The listing builds one solid part. Answer for the finished solid, in the listing's coordinates (mm). Face numbers are marked on the shaded views. A direction names the side the tool comes from. Round coordinates to 2 decimals unless told otherwise and drop trailing zeros. Loops run counter-clockwise (first coordinate to the right, second up) from the corner with the lowest first, then second, coordinate; pieces in that order, holes last. Notation, with made-up numbers: (81.5, 54.5) - (102.5, 54.5) arc R16 cw to (102.5, 79.5) - close; hole circle Ø1 at (-25, 82.25). An arc over 180 degrees is marked (long way). One line per item, written item: value.
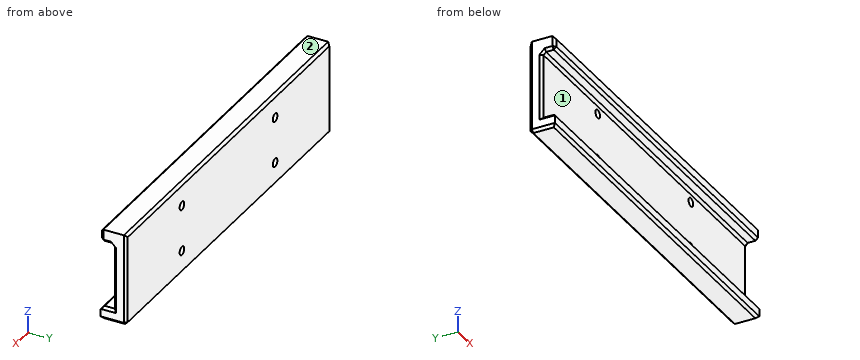
```python
from build123d import *

# Parameters (mm, degrees)
SKETCH1_W                       = 147
SKETCH1_H                       = 36
BOSS_EXTRUDE1_DEPTH             = 5
SKETCH2_W                       = 26
SKETCH2_H                       = 5
CUT_EXTRUDE1_DEPTH              = 74.5
CUT_EXTRUDE1_DEPTH_BACK         = 74.5
CHAMFER1_SIZE                   = 1
TAP_DRILL_FOR_M4X0_7_TAP1_D     = 3.3
TAP_DRILL_FOR_M4X0_7_TAP1_DEPTH = 14
TAP_DRILL_FOR_M4X0_7_TAP1_TIP   = 0.991420021


with BuildPart() as part:
    # Sketch1 → Boss-Extrude1 (new body, symmetric)
    with BuildSketch(Plane(origin=(0, 0, 0), x_dir=(1, 0, 0), z_dir=(0, 1, 0))):
        Rectangle(SKETCH1_W, SKETCH1_H)
    extrude(amount=BOSS_EXTRUDE1_DEPTH, both=True)

    # Sketch2 → Cut-Extrude1 (cut, two sides)
    with BuildSketch(Plane(origin=(0, 0, 0), x_dir=(0, 0, -1), z_dir=(1, 0, 0))) as cut_extrude1_sk:
        with Locations((0, -2.5)):
            Rectangle(SKETCH2_W, SKETCH2_H)
    extrude(amount=CUT_EXTRUDE1_DEPTH, mode=Mode.SUBTRACT)
    extrude(cut_extrude1_sk.sketch, amount=-CUT_EXTRUDE1_DEPTH_BACK, mode=Mode.SUBTRACT)

    # Chamfer1
    chamfer1_edges = [part.edges().sort_by_distance(p)[0] for p in [
        (73.5, -2.5, 13),
        (0, -5, 18),
        (0, 0, 13),
        (73.5, 0, 0),
        (73.5, -2.5, -13),
        (0, -5, -13),
        (-73.5, -2.5, -13),
        (-73.5, 0, 0),
        (-73.5, -2.5, 13),
        (-73.5, -5, 15.5),
        (0, -5, 13),
        (73.5, -5, 15.5),
        (0, 5, 18),
        (-73.5, 5, 0),
        (73.5, 5, 0),
        (0, 5, -18),
        (73.5, 0, -18),
        (0, -5, -18),
        (-73.5, 0, -18),
    ]]
    chamfer(chamfer1_edges, length=CHAMFER1_SIZE)

    # Tap Drill for M4x0.7 Tap1
    with Locations(Plane(origin=(-88.5, 5, -18), x_dir=(-1, 0, 0), z_dir=(0, 1, 0))):
        with Locations((-55, 27), (-122, 27), (-55, 9), (-122, 9)):
            Hole(TAP_DRILL_FOR_M4X0_7_TAP1_D / 2, depth=TAP_DRILL_FOR_M4X0_7_TAP1_DEPTH)
            with Locations((0, 0, -(TAP_DRILL_FOR_M4X0_7_TAP1_DEPTH + TAP_DRILL_FOR_M4X0_7_TAP1_TIP / 2))):  # 118° drill point
                Cone(0, TAP_DRILL_FOR_M4X0_7_TAP1_D / 2, TAP_DRILL_FOR_M4X0_7_TAP1_TIP, mode=Mode.SUBTRACT)


solid = part.part
```
1) For the marked faces 1 and 2, determine the directions among +Z, -Z, +X, -X, +Y, -Y from which every point of the face is accessible in a straight line to the end or side of a thin tool.
Final values:
face 1: +X, -X, -Y
face 2: +Z, +X, -X, +Y, -Y
2) Each of these flat-tipped pins is pushed along its axis until it touches: pin 1 Ø2.5 at (x, z) = (33.5, 9) entering from +Y; pin 2 Ø4 at (x, z) = (-33.5, -9) entering from -Y. Where does it stop, or does it pass through?
Final values:
pin 1: through
pin 2: y = 0
3) A cutting plane is placed at A-A on z = -9. Give the vertices of the cut face in (x, y).
Final values:
outline: (-73.5, 1) - (-72.5, 0) - (-35.15, 0) - (-35.15, 5) - (-72.5, 5) - (-73.5, 4) - close; (-31.85, 0) - (31.85, 0) - (31.85, 5) - (-31.85, 5) - close; (35.15, 0) - (72.5, 0) - (73.5, 1) - (73.5, 4) - (72.5, 5) - (35.15, 5) - close
4) Consider L1, parallel to Z at x = -33.5, y = 3; L2, parallel to Z at x = 54, y = -1.75; L3, parallel to Y at x = -49.5, z = -6.5. Determine where each line is inside the solid, lowest interval first.
Final values:
L1: -18 to -10.65, -7.35 to 7.35, 10.65 to 18
L2: -18 to -13, 13 to 18
L3: 0 to 5
5) A cutting plane is placed at B-B on x = -33.5. Give the vertices of the cut face in (y, z).
Final values:
outline: (-5, -17) - (-4, -18) - (4, -18) - (5, -17) - (5, -10.65) - (0, -10.65) - (0, -13) - (-4, -13) - (-5, -14) - close; (-5, 14) - (-4, 13) - (-1, 13) - (0, 12) - (0, 10.65) - (5, 10.65) - (5, 17) - (4, 18) - (-4, 18) - (-5, 17) - close; (0, -7.35) - (5, -7.35) - (5, 7.35) - (0, 7.35) - close
